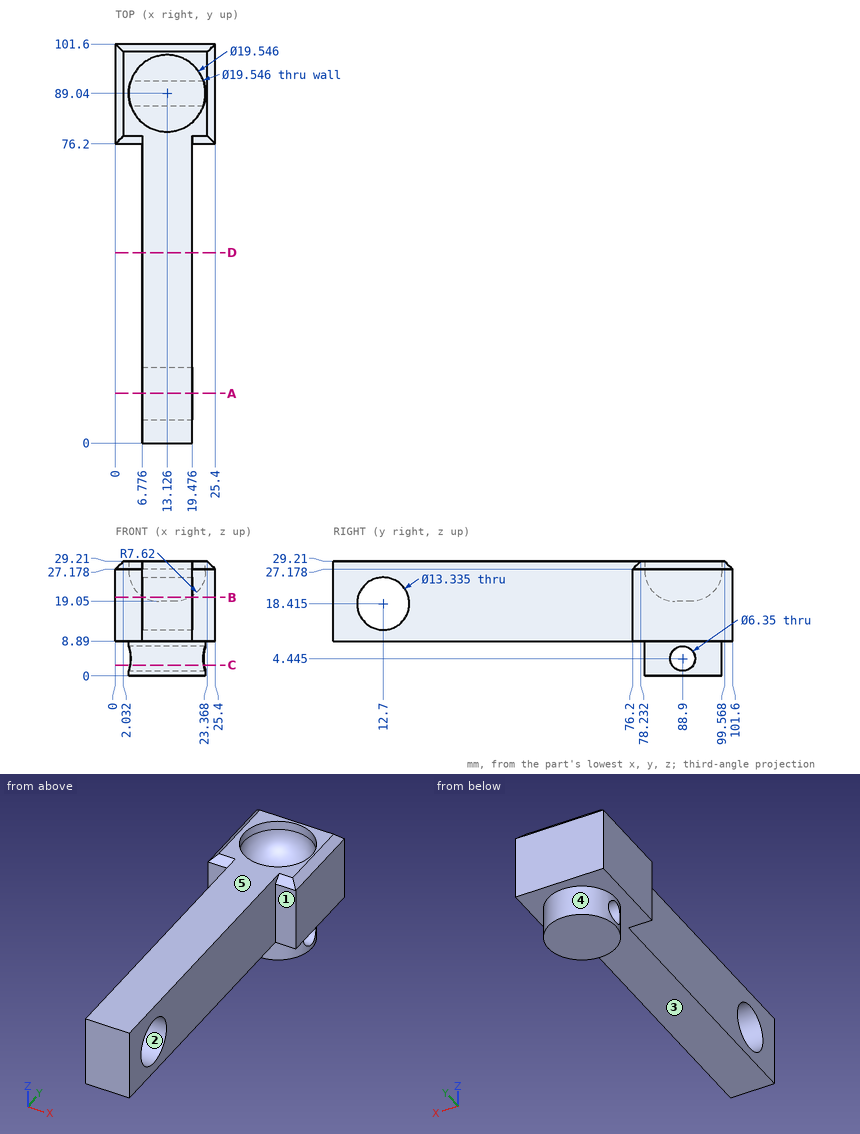
For this review, use the dimensioned drawing (mm, ordinates from the lowest corner) and the shaded views. A direction names the side the tool comes from. Coordinates: 2 decimals unless noted, no trailing zeros. Loops run counter-clockwise (first coordinate to the right, second up) from the corner with the lowest first, then second, coordinate; pieces in that order, holes last. Notation, with made-up numbers: M -29.5,83 L -5.5,83 A15 ccw -5.5,99 Z; hole C 44.25,75.25 d9. An arc over 180 degrees is marked long. Answer as CSV lines item,"result".
Item 1: For P1, Ø1, axis at y = 55, z = 20.5, coming from the +X side; P2, Ø8, axis at y = 42.5, z = 23, coming from the -X side; P3, Ø8, axis at y = 12.7, z = 18.415, coming from the +X side; P4, Ø5, axis at x = 15, y = 14.5, coming from the -Z side, all flat-tipped, find the tip position at first contact; note any pin that passes through.
Answer list:
P1,"x = 19.48"
P2,"x = 6.78"
P3,"through"
P4,"z = 8.89"
Item 2: Add section A-A on y = 12.7. State the section outline as (x, z) points (1 decimal).
Answer list:
outline,"M 6.8,8.9 L 19.5,8.9 L 19.5,11.7 L 6.8,11.7 Z; M 6.8,25.1 L 19.5,25.1 L 19.5,29.2 L 6.8,29.2 Z"
Item 3: Add section C-C on z = 2.75. State the section outline as (x, y) points (1 decimal).
Answer list:
outline,"M 3.7,91.6 L 22.6,91.6 A9.8 ccw Z; M 3.8,86.2 A9.8 ccw 22.5,86.2 Z"
Item 4: Add section D-D on y = 48.5. State the section outline as (x, z) points (1 decimal).
Answer list:
outline,"M 6.8,8.9 L 19.5,8.9 L 19.5,29.2 L 6.8,29.2 Z"
Item 5: Add section B-B on z = 20. Count the separate pieces of the cut face and the enclosed holes in it, plus the area to 3 significant figures.
Answer list:
separate pieces,"2"
enclosed holes,"1"
area,"1,340 mm²"
Item 6: For probe 1 along Z at (x, y) = (13.75, 88.9); probe 2 along Y at (x, z) = (15.5, 18.75); probe 3 along Y at (x, z) = (11.25, 22.5), list the stretches that pass through material, from the lowest coordinate up.
Answer list:
probe 1,"0 to 1.27, 7.62 to 19.05"
probe 2,"0 to 6.04, 19.36 to 101.6"
probe 3,"0 to 7.43, 17.97 to 80.72, 97.36 to 101.6"
Item 7: The part is to be moulded in two halves that separate along Y. For the marked faces 1, 2 and 3, say which applies: pulls with the +Y half, pulls with the -Y half, needs draft (parallel to the pull), parting line crosses it, or undercut.
Answer list:
face 1,"pulls with the -Y half"
face 2,"undercut"
face 3,"needs draft"
Item 8: Machinability: for the marked faces 4 and 5, which of the approach directions +Z, -Z, +X, -X, +Y, -Y give a long, thin tool a straight path to every point of the face, cutting with its end or side? Answer none if there is none.
Answer list:
face 4,"-Z"
face 5,"+Z, +X, -X, +Y, -Y"
